The drawing under review shows one solid part. Ordinate dimensions are in mm from its lowest x, y, z. Give positions to 0.01 mm unless a question says otherwise; leave off trailing zeros. Order: outer loops, then holes, each group sorted by start corner. A loop starts at its lowest first (then second) coordinate and runs counter-clockwise, first axis right, second up. Notation, with made-up numbers: M 88,43 L 102,43 A26 cw 102,67 Z; hole C 74,36 d2. An arc over 180 degrees is marked long. Put each result on its own line as item: value. Start each with the question number.
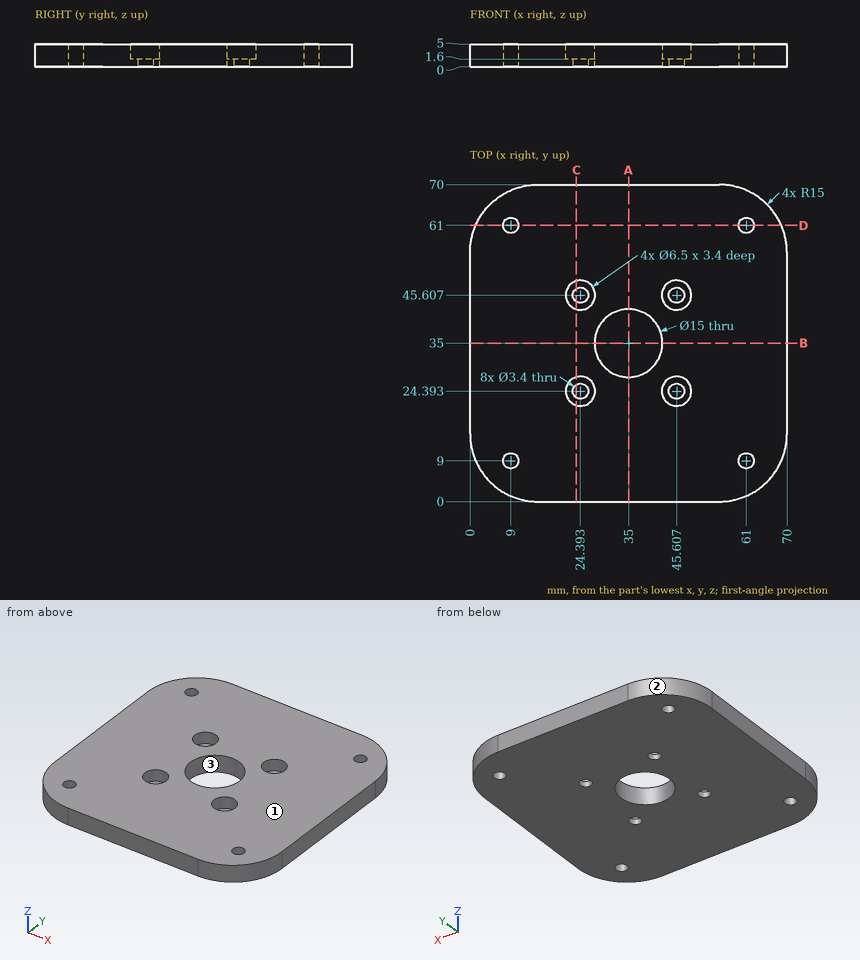
1. Insertion check: pin 1 (4.5 mm diameter, centred on x = 24.39, y = 45.61, fed in from +Z); pin 2 (3 mm diameter, centred on y = 13, z = 4, fed in from -X). Each pin has a flat end and moves straight along its axis. Give the tip position at first contact, or say it passes through.
2. Consider section D-D on y = 61. Give the boundary of the cut face in (x, z).
3. Consider section C-C on x = 23.5. Give the boundary of the cut face in (y, z).
4. The part is to be moulded in two halves that separate along X. For the marked faces 1, 2 and 3, say which applies: +X half, -X half, draft (parallel to the pull), parting line (faces both ways), or undercut.
5. Consider section A-A on x = 35. Give the boundary of the cut face in (y, z), then the cut area to 3 significant figures.
6. To check wall thickness, follow probe 1 along Y at (x, z) = (33.5, 3.05); probe 2 along Y at (x, z) = (23.5, 0.5); probe 3 along Y at (x, z) = (61, 2.7). State the ranges of each line that lie inside material, in increasing order.
Returned:
1. pin 1: stops at z = 1.6
1. pin 2: stops at x = 0.01
2. outline: M 1.25,0 L 7.3,0 L 7.3,5 L 1.25,5 Z; M 10.7,0 L 59.3,0 L 59.3,5 L 10.7,5 Z; M 62.7,0 L 68.75,0 L 68.75,5 L 62.7,5 Z
3. outline: M 0,0 L 22.95,0 L 22.95,1.6 L 21.27,1.6 L 21.27,5 L 0,5 Z; M 25.84,0 L 44.16,0 L 44.16,1.6 L 42.48,1.6 L 42.48,5 L 27.52,5 L 27.52,1.6 L 25.84,1.6 Z; M 47.05,0 L 70,0 L 70,5 L 48.73,5 L 48.73,1.6 L 47.05,1.6 Z
4. face 1: draft
4. face 2: -X half
4. face 3: undercut
5. outline: M 0,0 L 27.5,0 L 27.5,5 L 0,5 Z; M 42.5,0 L 70,0 L 70,5 L 42.5,5 Z
5. area: 275 mm2
6. probe 1: y = 0 to 27.65, 42.35 to 70
6. probe 2: y = 0 to 22.95, 25.84 to 44.16, 47.05 to 70
6. probe 3: y = 1.25 to 7.3, 10.7 to 59.3, 62.7 to 68.75
